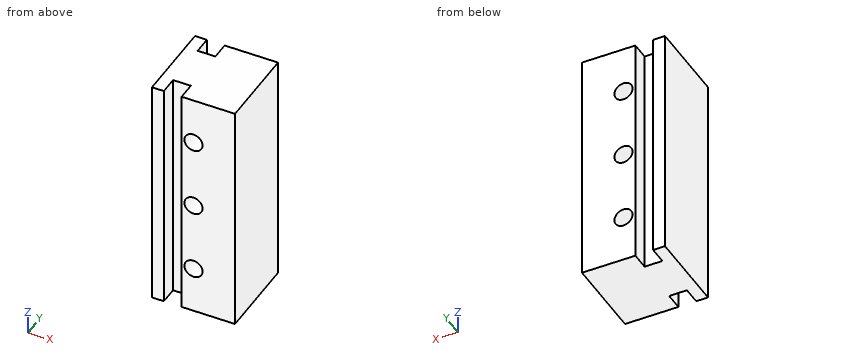
Autodesk Inventor part; units mm, degrees
ref_plane "YZ Plane" through (0, 0, 0) normal (1, 0, 0) x (0, 1, 0)
ref_plane "XZ Plane" through (0, 0, 0) normal (0, 1, 0) x (-1, 0, 0)
ref_plane "XY Plane" through (0, 0, 0) normal (0, 0, 1) x (1, 0, 0)
sketch "Sketch1" plane through (0, 0, 0) normal (0, 0, 1) x (1, 0, 0)
  line L0 (0, 0) -> (22.225, 0)
  line L1 (22.225, 0) -> (22.225, 22.225)
  line L2 (22.225, 22.225) -> (0, 22.225)
  line L3 (0, 22.225) -> (0, 0)
  dimension "d0" = 22.225
extrude "Extrusion1" add sketch "Sketch1" along normal blind 63.5
sketch "Sketch2" plane through (0, 22.225, 0) normal (0, 1, 0) x (1, 0, 0)
  line L0 (0, 0) -> (0, -63.5)
  line L1 (22.225, -63.5) -> (0, -63.5)
  line L2 (22.225, 0) -> (0, 0)
  point P0 (11.1125, -12.7)
  point P1 (11.1125, -31.75)
  point P2 (11.1125, -50.8)
  point P3 (11.1125, 0)
  dimension "d26" = 12.7
  dimension "d28" = 19.05
  dimension "d29" = 19.05
hole "Hole1" at (11.1125, 22.225, 12.7) at (11.1125, 22.225, 31.75) at (11.1125, 22.225, 50.8) direction (0, -1, 0) diameter 4.8514 end through all
sketch "Sketch3" plane through (0, 0, 63.5) normal (0, 0, 1) x (1, 0, 0)
  line L0 (22.225, 22.225) -> (0, 22.225)
  line L1 (22.225, 0) -> (22.225, 22.225)
  line L2 (0, 22.225) -> (0, 0)
  line L3 (0, 0) -> (22.225, 0)
  point P0 (4.7625, 17.4625)
  point P1 (4.7625, 4.7625)
  dimension "d21" = 4.7625
  dimension "d22" = 4.7625
  dimension "d31" = 4.7625
hole "Hole2" [suppressed]
sketch "Sketch4" plane through (0, 0, 63.5) normal (0, 0, 1) x (1, 0, 0)
  line L0 (3.175, 27.2947) -> (7.9375, 27.2947)
  line L1 (7.9375, 27.2947) -> (7.9375, 17.4625)
  line L2 (7.9375, 17.4625) -> (3.175, 17.4625)
  line L3 (3.175, 17.4625) -> (3.175, 27.2947)
  line L4 (3.175, -4.5253) -> (7.9375, -4.5253)
  line L5 (7.9375, -4.5253) -> (7.9375, 4.7625)
  line L6 (7.9375, 4.7625) -> (3.175, 4.7625)
  line L7 (3.175, 4.7625) -> (3.175, -4.5253)
  line L8 (0, 0) -> (22.225, 0)
  line L9 (22.225, 22.225) -> (0, 22.225)
  line L10 (0, 22.225) -> (0, 0)
  dimension "d32" = 4.7625
  dimension "d33" = 4.7625
  dimension "d34" = 4.7625
  dimension "d35" = 7.9375
  dimension "d38" = 3.175
extrude "Extrusion2" cut sketch "Sketch4" against normal through all
equation "\"d34\" = d33"
properties part number "CLB_052_ScissorLiftPlug" material "Nylon 6/6"
Check sheet for the modelled part. Datum: model origin and axes. Units: mm. Round coordinates to 2 decimals unless told otherwise and drop trailing zeros. Order: outer loops, then holes, each group sorted by start corner. A loop starts at its lowest first (then second) coordinate and runs counter-clockwise, first axis right, second up.
1) Go/stop test with a flat-tipped pin: pin 1 Ø1 at (x, y) = (4.5, 2) entering from -Z. Record where the tip stops, or that it passes through.
2) Scan lines: line 1 (X direction, y = 12.25, z = 31.75) (3 decimals); line 2 (X direction, y = 19.25, z = 49) (1 decimal); line 3 (X direction, y = 3, z = 28.5) (1 decimal). Record each from-to range of solid material in increasing order.
3) Section check A-A (y = 18.25). Give the number of separate pieces and of enclosed holes in the cut face, and give its area (3 significant figures).
4) Section check C-C (x = 6). Record the boundary of the cut face in (y, z), and give its area (3 significant figures).
5) Section check B-B (z = 31.75). Record the boundary of the cut face in (x, y) (1 decimal), and give its area (3 significant figures).
Result:
1. pin 1: passes through
2. line 1: x = 0 to 8.687, 13.538 to 22.225
2. line 2: x = 0 to 3.2, 7.9 to 9.5, 12.7 to 22.2
2. line 3: x = 0 to 3.2, 7.9 to 22.2
3. separate pieces: 2
3. enclosed holes: 3
3. area: 1,050 mm2
4. outline: (4.76, 0) - (17.46, 0) - (17.46, 63.5) - (4.76, 63.5) - close
4. area: 806 mm2
5. outline: (0, 0) - (3.2, 0) - (3.2, 4.8) - (7.9, 4.8) - (7.9, 0) - (8.7, 0) - (8.7, 22.2) - (7.9, 22.2) - (7.9, 17.5) - (3.2, 17.5) - (3.2, 22.2) - (0, 22.2) - close; (13.5, 0) - (22.2, 0) - (22.2, 22.2) - (13.5, 22.2) - close
5. area: 341 mm2
